Can you work these out from the drawing? Everything is in mm from the part's minimum corner. A direction names the side the tool comes from. Round coordinates to 2 decimals unless told otherwise and drop trailing zeros. Loops run counter-clockwise (first coordinate to the right, second up) from the corner with the lowest first, then second, coordinate; pieces in that order, holes last. Notation, with made-up numbers: M 1.5,77 L 15.5,77 A20 ccw 15.5,81 Z; hole C 1.5,73 d9. An arc over 180 degrees is marked long. Use a Markdown table: item, result.
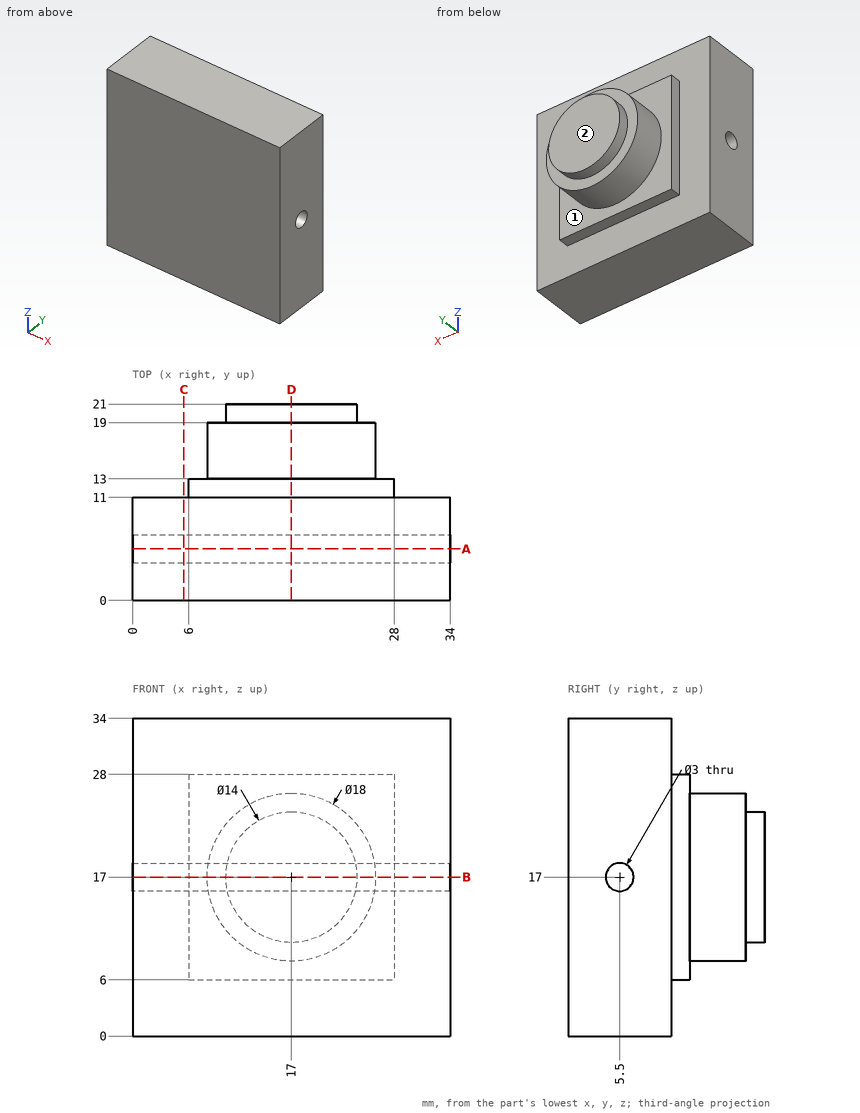
Q1. Imagine slicing it at A-A, the plane y = 5.5. Please give me the cut outline in (x, z).
Return value:
| item | result |
|---|---|
| outline | M 0,0 L 34,0 L 34,15.5 L 0,15.5 Z; M 0,18.5 L 34,18.5 L 34,34 L 0,34 Z |
Q2. Imagine slicing it at D-D, the plane x = 17. Please give me the cut outline in (y, z).
Return value:
| item | result |
|---|---|
| outline | M 0,0 L 11,0 L 11,6 L 13,6 L 13,8 L 19,8 L 19,10 L 21,10 L 21,24 L 19,24 L 19,26 L 13,26 L 13,28 L 11,28 L 11,34 L 0,34 Z; hole C 5.5,17 d3 |
Q3. For the marked faces 1 and 2, which set-ups out of +Z, -Z, +X, -X, +Y, -Y let a thin tool reach every point of the face, with its end or its side?
Return value:
| item | result |
|---|---|
| face 1 | +Y |
| face 2 | +Z, -Z, +X, -X, +Y |
Q4. I need wall thicknesses on line 1 (Y direction, x = 25, z = 17); line 2 (Y direction, x = 27.5, z = 17); line 3 (Y direction, x = 28.5, z = 24.5). Which ranges of each line are inside material? Lowest first, please. Write a range as from..to.
Return value:
| item | result |
|---|---|
| line 1 | y = 0..4, 7..19 |
| line 2 | y = 0..4, 7..13 |
| line 3 | y = 0..11 |
Q5. Imagine slicing it at C-C, the plane x = 5.5. Please give me the cut outline in (y, z).
Return value:
| item | result |
|---|---|
| outline | M 0,0 L 11,0 L 11,34 L 0,34 Z; hole C 5.5,17 d3 |
Q6. Imagine slicing it at B-B, the plane z = 17. Please give me the cut outline in (x, y).
Return value:
| item | result |
|---|---|
| outline | M 0,0 L 34,0 L 34,4 L 0,4 Z; M 0,7 L 34,7 L 34,11 L 28,11 L 28,13 L 26,13 L 26,19 L 24,19 L 24,21 L 10,21 L 10,19 L 8,19 L 8,13 L 6,13 L 6,11 L 0,11 Z |
Q7. Will these pins go through, and if not, where does the flat tip stop? P1, Ø1.6, axis at x = 19.5, y = 12, coming from the -Z side; P2, Ø0.6, axis at x = 19, y = 12, coming from the +Z side; P3, Ø1, axis at x = 27.5, y = 17, coming from the -Z side; P4, Ø3, axis at y = 13, z = 6.5, coming from the -X side.
Return value:
| item | result |
|---|---|
| P1 | stops at z = 6 |
| P2 | stops at z = 28 |
| P3 | passes through |
| P4 | stops at x = 6 |
